Work out the finished part from the listing and answer in its coordinate system (mm). A direction names the side the tool comes from. Coordinates: 2 decimals unless noted, no trailing zeros. Order: outer loops, then holes, each group sorted by start corner. A loop starts at its lowest first (then second) coordinate and runs counter-clockwise, first axis right, second up. Notation, with made-up numbers: M 34,51 L 50,51 A7 ccw 50,56 Z; hole C 7.25,65.5 d11. An arc over 180 degrees is marked long. Use a Markdown table: item, result.
from build123d import *

# Parameters (mm, degrees)
F1_DEPTH = 3.175
F0_R     = 3.8862
F2_DEPTH = 4.7498
F3_R     = 2.3495
F4_DEPTH = 76.2


with BuildPart() as f1:
    # F0 (on Front) → F1 (new body)
    with BuildSketch(Plane.XZ):
        Polygon((1.869749, -1.0795), (1.869749, 1.0795), (0, 2.159), (-1.869749, 1.0795), (-1.869749, -1.0795), (0, -2.159), align=None)
    extrude(amount=F1_DEPTH)

    # F0 (on Front) → F2 (join)
    with BuildSketch(Plane.XZ):
        Circle(F0_R)
        Polygon((0, 2.159), (1.869749, 1.0795), (1.869749, -1.0795), (0, -2.159), (-1.869749, -1.0795), (-1.869749, 1.0795), align=None, mode=Mode.SUBTRACT)
    extrude(amount=F2_DEPTH)

    # F3 (on face) → F4 (join)
    with BuildSketch(Plane(origin=(0, 0, 0), x_dir=(-1, 0, 0), z_dir=(0, 1, 0))):
        Circle(F3_R)
    extrude(amount=F4_DEPTH)


solid = f1.part
(1) Given P1, Ø0.5, axis at y = -4, z = -0.5, coming from the -X side; P2, Ø1.7, axis at y = -4, z = -0.5, coming from the +X side; P3, Ø1, axis at x = -2.5, y = 20.5, coming from the +Z side; P4, Ø3, axis at x = 3, y = 14.5, coming from the -Z side, each flat-ended and moving along its own axis, determine where each tip first touches the part or whether it passes through.
Conclusion:
| item | result |
|---|---|
| P1 | x = -3.88 |
| P2 | x = 3.89 |
| P3 | z = 1.23 |
| P4 | z = -1.81 |
(2) Which of the six approach directions +Z, -Z, +X, -X, +Y, -Y give full straight-line access (tool end or side, diameter ignored) to faces 1 (the flat face through (0, -3.175, 0)), 2 (the flat face through (-1, -4.75, -2)), 3 (the cylindrical face through (0.31, 37.57, 2.33))?
Conclusion:
| item | result |
|---|---|
| face 1 | -Y |
| face 2 | +Z, -Z, +X, -X, -Y |
| face 3 | +Y |
(3) A cutting plane is placed at B-B (x = 1). Determine the outline of the cut face in (y, z) (3 decimals).
Conclusion:
| item | result |
|---|---|
| outline | M -4.75,-3.755 L 0,-3.755 L 0,-2.126 L 76.2,-2.126 L 76.2,2.126 L 0,2.126 L 0,3.755 L -4.75,3.755 L -4.75,1.582 L -3.175,1.582 L -3.175,-1.582 L -4.75,-1.582 Z |
(4) A cutting plane is placed at A-A (z = 0). Determine the outline of the cut face in (x, y) (1 decimal), then the cut area to 3 significant figures.
Conclusion:
| item | result |
|---|---|
| outline | M -3.9,-4.7 L -1.9,-4.7 L -1.9,-3.2 L 1.9,-3.2 L 1.9,-4.7 L 3.9,-4.7 L 3.9,0 L 2.3,0 L 2.3,76.2 L -2.3,76.2 L -2.3,0 L -3.9,0 Z |
| area | 389 mm2 |
(5) Straight lines are drawn through the part: L1, parallel to Y at x = 1.25, z = 0.75 (3 decimals); L2, parallel to Y at x = -1, z = -2.75; L3, parallel to Z at x = -0.25, y = 4.5. For each, find the intervals that lie inside material, in ascending order.
Conclusion:
| item | result |
|---|---|
| L1 | -3.175 to 76.2 |
| L2 | -4.75 to 0 |
| L3 | -2.34 to 2.34 |
(6) Determine the mould class of faces 4 (the flat face through (-0.95, -3.95, 1.61)), 5 (the cylindrical face through (3.707, -2.342, 1.167)), 6 (the flat face through (0, 76.2, 0)) for opening direction X: pulls with the +X half, pulls with the -X half, needs draft (parallel to the pull), parting line crosses it, or undercut.
Conclusion:
| item | result |
|---|---|
| face 4 | undercut |
| face 5 | parting line crosses it |
| face 6 | needs draft |
(7) A cutting plane is placed at C-C (y = 61). Determine the outline of the cut face in (x, z), then the cut area to 3 significant figures.
Conclusion:
| item | result |
|---|---|
| outline | C 0,0 d4.7 |
| area | 17.3 mm2 |
